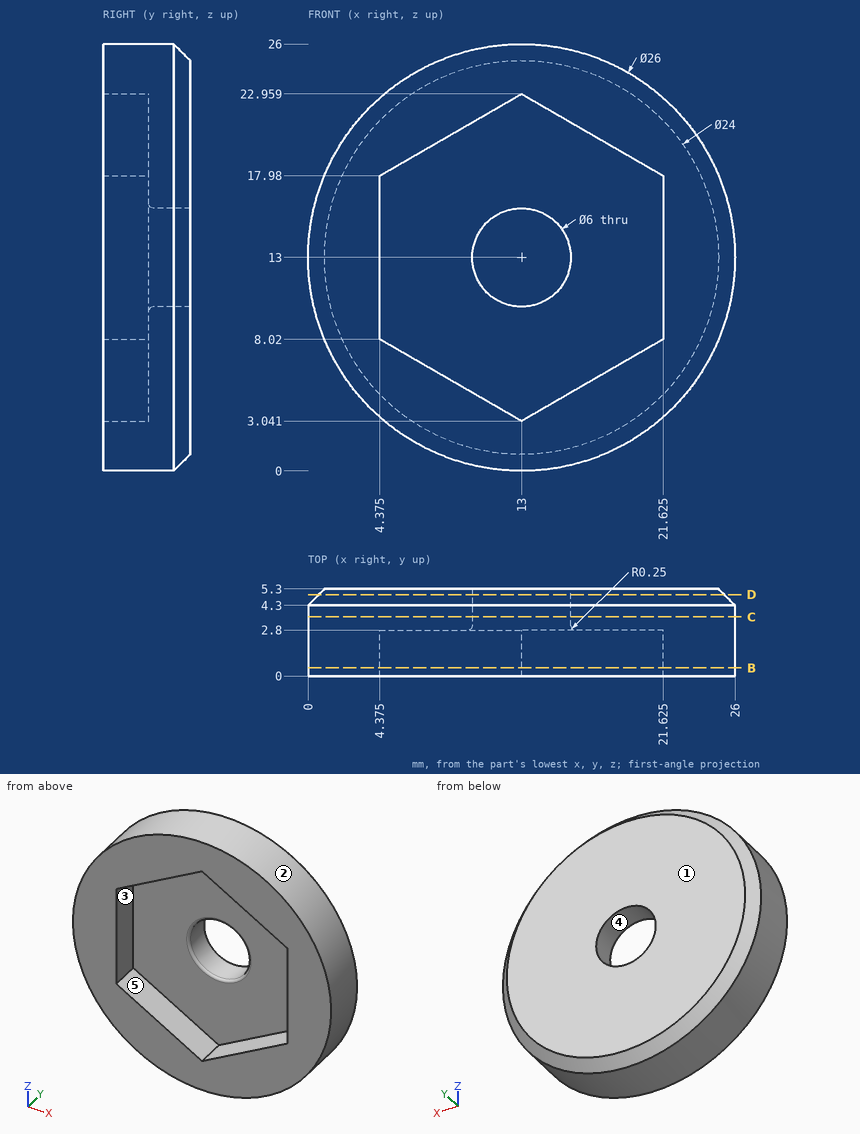
For this review, use the dimensioned drawing (mm, ordinates from the lowest corner) and the shaded views. A direction names the side the tool comes from. Round coordinates to 2 decimals unless told otherwise and drop trailing zeros. Order: outer loops, then holes, each group sorted by start corner. A loop starts at its lowest first (then second) coordinate and runs counter-clockwise, first axis right, second up. Notation, with made-up numbers: (-33, 71.5) -> (-9, 71.5) arc R19 ccw to (-9, 107.5) -> close; hole circle Ø3 at (0, -2.75). An arc over 180 degrees is marked (long way). Use CSV: the item, a comma, the result in double quotes. Start each with the question number.
(1) Consider section B-B on y = 0.5. Write out the cut boundary in (x, z) (1 decimal), and give its area (3 significant figures).
(2) Consider section C-C on y = 3.6. Write out the cut boundary in (x, z), and give its area (3 significant figures).
(3) Insertion check: pin 1 (1 mm diameter, centred on x = 9.5, y = 2.5, fed in from +Z); pin 2 (2 mm diameter, centred on y = 1, z = 15, fed in from +X); pin 3 (9.5 mm diameter, centred on x = 13, z = 13, fed in from -Y). Each pin has a flat end and moves straight along its axis. Give the tip position at first contact, or say it passes through.
(4) Wall thickness on probe 1 along X at (y, z) = (4.15, 13); probe 2 along Y at (x, z) = (18.25, 18); probe 3 along Z at (x, y) = (9.5, 0.7): over which ranges is each line inside the solid? List them lowest first. Write a range as from..to.
(5) Consider section D-D on y = 4.95. Write out the cut boundary in (x, z), and give its area (3 significant figures).
(6) Tool access review of the marked faces 4 and 5: name each direction out of +Z, -Z, +X, -X, +Y, -Y from which nothing blocks a thin tool from reaching the whole face with its end or side.
(7) Mouldability with a two-part tool opening along X and no side actions: class the marked faces 1, 2 and 3 as pulls with the +X half, pulls with the -X half, needs draft (parallel to the pull), parting line crosses it, or undercut.
Responses:
1,outline,"circle Ø26 at (13, 13); hole (4.4, 8) -> (13, 3) -> (21.6, 8) -> (21.6, 18) -> (13, 23) -> (4.4, 18) -> close"
1,area,"273 mm²"
2,outline,"circle Ø26 at (13, 13); hole circle Ø6 at (13, 13)"
2,area,"503 mm²"
3,pin 1,"z = 25.65"
3,pin 2,"x = 25.96"
3,pin 3,"y = 2.8"
4,probe 1,"0..10, 16..26"
4,probe 2,"2.8..5.3"
4,probe 3,"0.48..5.06, 20.94..25.52"
5,outline,"circle Ø24.7 at (13, 13); hole circle Ø6 at (13, 13)"
5,area,"451 mm²"
6,face 4,"+Y, -Y"
6,face 5,"-Y"
7,face 1,"needs draft"
7,face 2,"parting line crosses it"
7,face 3,"undercut"
